```python
from build123d import *

# Parameters (mm, degrees)
Y_KSEKLIK_EKSTR_ZYON1_DEPTH = 13
Y_KSEKLIK_EKSTR_ZYON2_DEPTH = 6.8
IZIM3_R                     = 1.25
KES_EKSTR_ZYON1_DEPTH       = 13.8


with BuildPart() as part:
    # Çizim1 → Yükseklik-Ekstrüzyon1 (new body)
    with BuildSketch(Plane.XY):
        Polygon((3.7, 0), (1.85, 3.204293994), (-1.85, 3.204293994), (-3.7, 0), (-1.85, -3.204293994), (1.85, -3.204293994), align=None)
    extrude(amount=Y_KSEKLIK_EKSTR_ZYON1_DEPTH)

    # Çizim2 → Yükseklik-Ekstrüzyon2 (add)
    with BuildSketch(Plane.XY.offset(13)):
        with BuildLine():
            Line((1.85, -3.204293994), (3.2, -3.204293994))
            ThreePointArc((3.2, -3.204293994), (3.553553391, -3.057847385), (3.7, -2.704293994))
            Line((3.7, -2.704293994), (3.7, -2))
            Line((3.7, -2), (3.7, 2.325966452))
            Line((3.7, 2.325966452), (3.7, 2.704293994))
            ThreePointArc((3.7, 2.704293994), (3.553553391, 3.057847385), (3.2, 3.204293994))
            Line((3.2, 3.204293994), (1.85, 3.204293994))
            Line((1.85, 3.204293994), (-1.85, 3.204293994))
            Line((-1.85, 3.204293994), (-3.2, 3.204293994))
            ThreePointArc((-3.2, 3.204293994), (-3.553553391, 3.057847385), (-3.7, 2.704293994))
            Line((-3.7, 2.704293994), (-3.7, 2.328172496))
            Line((-3.7, 2.328172496), (-3.7, -2))
            Line((-3.7, -2), (-3.7, -2.704293994))
            ThreePointArc((-3.7, -2.704293994), (-3.553553391, -3.057847385), (-3.2, -3.204293994))
            Line((-3.2, -3.204293994), (-1.85, -3.204293994))
            Line((-1.85, -3.204293994), (1.85, -3.204293994))
        make_face()
        with BuildLine():
            Line((-2.2, -1.8), (2.2, -1.8))
            ThreePointArc((2.2, -1.8), (2.553553391, -1.653553391), (2.7, -1.3))
            Line((2.7, -1.3), (2.7, 1.3))
            ThreePointArc((2.7, 1.3), (2.553553391, 1.653553391), (2.2, 1.8))
            Line((2.2, 1.8), (-2.2, 1.8))
            ThreePointArc((-2.2, 1.8), (-2.553553391, 1.653553391), (-2.7, 1.3))
            Line((-2.7, 1.3), (-2.7, -1.3))
            ThreePointArc((-2.7, -1.3), (-2.553553391, -1.653553391), (-2.2, -1.8))
        make_face(mode=Mode.SUBTRACT)
    extrude(amount=Y_KSEKLIK_EKSTR_ZYON2_DEPTH)

    # Çizim3 → Kes-Ekstrüzyon1 (cut)
    with BuildSketch(Plane(origin=(0, 0, 0), x_dir=(-1, 0, 0), z_dir=(0, 0, -1))):
        Circle(IZIM3_R)
    extrude(amount=-KES_EKSTR_ZYON1_DEPTH, mode=Mode.SUBTRACT)


solid = part.part
```
CAD build for the part. Positions are in the model's coordinates, mm. A direction names the side the tool comes from. Round coordinates to 2 decimals unless told otherwise and drop trailing zeros. Write each loop counter-clockwise with the first axis right and the second up, starting at its lowest first coordinate (ties: lowest second). Pieces come first, ordered by that corner, then holes. Notation, with made-up numbers: (21, -31.5) -> (66, -31.5) arc R13 cw to (66, -23.5) -> close; hole circle Ø4 at (84.5, 59). An arc over 180 degrees is marked (long way). Answer in a Markdown table with one row per item. Add a question column.
Item 1: Saw through at D-D, the plane x = 2.5. Write the cut outline in (y, z).
Item 2: Saw through at C-C, the plane y = 1. Write the cut outline in (x, z).
Item 3: Saw through at B-B, the plane z = 16.25. Write the cut outline in (x, y).
Item 4: Mould opens along X. For faces 1 (the face through (-3, 2, 13)), 2 (the face through (2.79, 1.58, 6.41)), 3 (the face through (2.7, 0, 16)) say: pulls with the +X half, pulls with the -X half, needs draft (parallel to the pull), parting line crosses it, or undercut.
Item 5: Drop flat-ended pins along their axis: pin 1 Ø1.1 at (x, y) = (0, -1) entering from +Z; pin 2 Ø1.5 at (x, y) = (0, 0) entering from -Z; pin 3 Ø2 at (x, y) = (2.5, 2.5) entering from -Z. Give the stop position or say it passes through.
Item 6: Which spindle directions (+Z, -Z, +X, -X, +Y, -Y) get a long thin tool onto all of the face, cutting with end or side? Do faces 4 (the face through (3, 2, 13)), 5 (the face through (-2.762, 1.625, 6.409)), 6 (the face through (3, -2, 13)), 7 (the face through (-1, -1, 13)), 8 (the face through (-3, -2, 13)). Say none if no direction does.
Item 7: Saw through at A-A, the plane x = 0. Write the cut outline in (y, z), then the cut area to 3 significant figures.
Item 8: Drill centre lines: line 1 (Y direction, x = 0, z = 5.5); line 2 (X direction, y = -1, z = 16.75); line 3 (Y direction, x = -0.75, z = 16.25). Where is each one in solid material? Low to high. Write a range as from..to.
Findings below:
| question | item | result |
|---|---|---|
| 1 | outline | (-3.2, 13) -> (-2.08, 13) -> (-2.08, 0) -> (2.08, 0) -> (2.08, 13) -> (3.2, 13) -> (3.2, 19.8) -> (1.7, 19.8) -> (1.7, 13) -> (-1.7, 13) -> (-1.7, 19.8) -> (-3.2, 19.8) -> close |
| 2 | outline | (-3.7, 13) -> (-3.12, 13) -> (-3.12, 0) -> (-0.75, 0) -> (-0.75, 13) -> (-2.7, 13) -> (-2.7, 19.8) -> (-3.7, 19.8) -> close; (0.75, 0) -> (3.12, 0) -> (3.12, 13) -> (3.7, 13) -> (3.7, 19.8) -> (2.7, 19.8) -> (2.7, 13) -> (0.75, 13) -> close |
| 3 | outline | (-3.7, -2.7) arc R0.5 ccw to (-3.2, -3.2) -> (3.2, -3.2) arc R0.5 ccw to (3.7, -2.7) -> (3.7, 2.7) arc R0.5 ccw to (3.2, 3.2) -> (-3.2, 3.2) arc R0.5 ccw to (-3.7, 2.7) -> close; hole (-2.7, -1.3) arc R0.5 ccw to (-2.2, -1.8) -> (2.2, -1.8) arc R0.5 ccw to (2.7, -1.3) -> (2.7, 1.3) arc R0.5 ccw to (2.2, 1.8) -> (-2.2, 1.8) arc R0.5 ccw to (-2.7, 1.3) -> close |
| 4 | face 1 | needs draft |
| 4 | face 2 | pulls with the +X half |
| 4 | face 3 | undercut |
| 5 | pin 1 | stops at z = 13 |
| 5 | pin 2 | passes through |
| 5 | pin 3 | stops at z = 0 |
| 6 | face 4 | -Z, +X, +Y |
| 6 | face 5 | -Z, -X, +Y |
| 6 | face 6 | -Z, +X, -Y |
| 6 | face 7 | +Z |
| 6 | face 8 | -Z, -X, -Y |
| 7 | outline | (-3.2, 0) -> (-1.25, 0) -> (-1.25, 13) -> (-1.8, 13) -> (-1.8, 19.8) -> (-3.2, 19.8) -> close; (1.25, 0) -> (3.2, 0) -> (3.2, 19.8) -> (1.8, 19.8) -> (1.8, 13) -> (1.25, 13) -> close |
| 7 | area | 69.9 mm^2 |
| 8 | line 1 | y = -3.2..-1.25, 1.25..3.2 |
| 8 | line 2 | x = -3.7..-2.7, 2.7..3.7 |
| 8 | line 3 | y = -3.2..-1.8, 1.8..3.2 |
